from build123d import *

# Parameters (mm, degrees)
SKETCH1_R           = 2.5
BOSS_EXTRUDE1_DEPTH = 175


with BuildPart() as part:
    # Sketch1 → Boss-Extrude1 (new, symmetric)
    with BuildSketch(Plane.XY):
        Polygon((3.9, -2.839339828), (6.560660172, -5.5), (8.200660172, -5.5), (8.200660172, -3.1), (9.3, -3.1), (10, -3.8), (10, -10), (3.8, -10), (3.1, -9.3), (3.1, -8.200660172), (5.5, -8.200660172), (5.5, -6.560660172), (2.839339828, -3.9), (-2.839339828, -3.9), (-5.5, -6.560660172), (-5.5, -8.200660172), (-3.1, -8.200660172), (-3.1, -9.3), (-3.8, -10), (-10, -10), (-10, -3.8), (-9.3, -3.1), (-8.200660172, -3.1), (-8.200660172, -5.5), (-6.560660172, -5.5), (-3.9, -2.839339828), (-3.9, 2.839339828), (-6.560660172, 5.5), (-8.200660172, 5.5), (-8.200660172, 3.1), (-9.3, 3.1), (-10, 3.8), (-10, 10), (-3.8, 10), (-3.1, 9.3), (-3.1, 8.200660172), (-5.5, 8.200660172), (-5.5, 6.560660172), (-2.839339828, 3.9), (2.839339828, 3.9), (5.5, 6.560660172), (5.5, 8.200660172), (3.1, 8.200660172), (3.1, 9.3), (3.8, 10), (10, 10), (10, 3.8), (9.3, 3.1), (8.200660172, 3.1), (8.200660172, 5.5), (6.560660172, 5.5), (3.9, 2.839339828), align=None)
        Circle(SKETCH1_R, mode=Mode.SUBTRACT)
    extrude(amount=BOSS_EXTRUDE1_DEPTH, both=True)


solid = part.part
Input: part model. Units: mm. Frame: model coordinates. A direction names the side the tool comes from. Give positions to 0.01 mm unless a question says otherwise; leave off trailing zeros. Use CSV: the item, a comma, the result in double quotes.
(1) Material intervals for L1, parallel to Y at x = 0, z = 31; L2, parallel to X at y = -8.5, z = 77; L3, parallel to X at y = 3.75, z = 18.5, sorted ascending. Write a range as [from, to].
Outcome:
L1,"y = [-3.9, -2.5], [2.5, 3.9]"
L2,"x = [-10, -3.1], [3.1, 10]"
L3,"x = [-9.95, -8.2], [-4.81, 4.81], [8.2, 9.95]"
(2) Pin query (flat end, axial travel): P1, Ø0.7, axis at y = 3.5, z = 26, coming from the +X side; P2, Ø3, axis at y = -0.5, z = 1.5, coming from the +X side; P3, Ø4, axis at y = 0, z = -24.5, coming from the -X side. Return the tip coordinate at first contact, or that it passes through.
Outcome:
P1,"stops at x = 10"
P2,"stops at x = 3.9"
P3,"stops at x = -3.9"
(3) Set-up query: faces 4 (the face through (-3.9, 0, 2)), 5 (the face through (7, -10, 2)), 6 (the face through (0, -3.9, 2)). Return all of +Z, -Z, +X, -X, +Y, -Y with unobstructed straight access to the full face (end or side cutting, diameter ignored); none if empty.
Outcome:
face 4,"+Z, -Z, -X"
face 5,"+Z, -Z, +X, -X, -Y"
face 6,"+Z, -Z, -Y"
(4) Pull-direction query (Y, two-part tool) for faces 1 (the face through (0, 3.9, 2)), 2 (the face through (-10, 7, 2)), 3 (the face through (3.9, 0, 2)); classes: pulls with the +Y half, pulls with the -Y half, needs draft (parallel to the pull), parting line crosses it, or undercut.
Outcome:
face 1,"pulls with the +Y half"
face 2,"needs draft"
face 3,"undercut"
